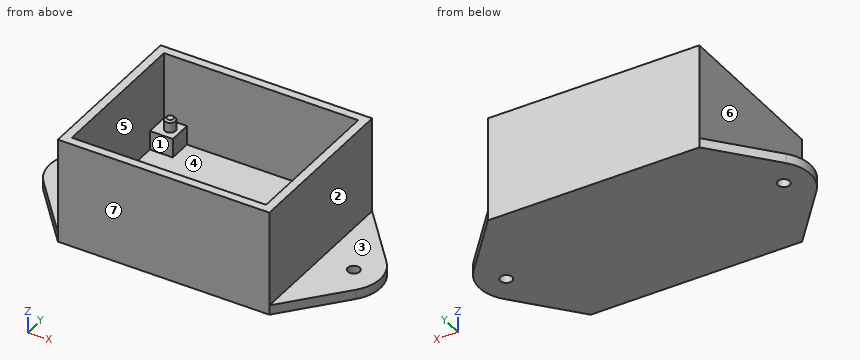
from build123d import *

# Parameters (mm, degrees)
F0_W      = 56.134
F0_H      = 44.45
F1_DEPTH  = 27.94
F2_W      = 51.562
F2_H      = 39.878
F3_DEPTH  = 22.86
F4_W      = 6.096
F4_H      = 6.096
F5_DEPTH  = 5.08
F6_R      = 1.397
F7_DEPTH  = 3.175
F8_SIZE   = 0.508
F10_DEPTH = 2.54
F11_R     = 1.5875
F12_DEPTH = 25.4


with BuildPart() as f1:
    # F0 (on Top) → F1 (new body)
    with BuildSketch(Plane.XY):
        Rectangle(F0_W, F0_H)
    extrude(amount=F1_DEPTH)

    # F2 (on face) → F3 (cut)
    with BuildSketch(Plane.XY.offset(27.94)):
        Rectangle(F2_W, F2_H)
    extrude(amount=-F3_DEPTH, mode=Mode.SUBTRACT)

    # F4 (on face) → F5 (join)
    with BuildSketch(Plane.XY.offset(5.08)):
        with Locations((-22.733, 16.891)):
            Rectangle(F4_W, F4_H)
        with Locations((22.733, 16.891)):
            Rectangle(F4_W, F4_H)
        with Locations((-22.733, -16.891)):
            Rectangle(F4_W, F4_H)
        with Locations((22.733, -16.891)):
            Rectangle(F4_W, F4_H)
    extrude(amount=F5_DEPTH)

    # F6 (on face) → F7 (join)
    with BuildSketch(Plane.XY.offset(10.16)):
        with Locations((-22.225, 16.85925)):
            Circle(F6_R)
        with Locations((22.225, 16.85925)):
            Circle(F6_R)
        with Locations((22.225, -16.85925)):
            Circle(F6_R)
        with Locations((-22.225, -16.85925)):
            Circle(F6_R)
    extrude(amount=F7_DEPTH)

    # F8
    f8_edges = [f1.edges().sort_by_distance(p)[0] for p in [
        (-23.622, 16.85925, 13.335),
        (20.828, 16.85925, 13.335),
        (-23.622, -16.85925, 13.335),
        (20.828, -16.85925, 13.335),
    ]]
    chamfer(f8_edges, length=F8_SIZE)

    # F9 (on face) → F10 (join)
    with BuildSketch(Plane(origin=(0, 0, 0), x_dir=(1, 0, 0), z_dir=(0, 0, -1))):
        with BuildLine():
            Line((41.449537, 6.61204), (28.067, 22.225))
            Line((28.067, 22.225), (28.067, -22.225))
            Line((28.067, -22.225), (41.449537, -6.61204))
            ThreePointArc((41.449537, -6.61204), (43.89549, 0), (41.449537, 6.61204))
        make_face()
        with BuildLine():
            Line((-28.067, -22.225), (-28.067, 22.225))
            Line((-28.067, 22.225), (-41.449537, 6.61204))
            ThreePointArc((-41.449537, 6.61204), (-43.89549, 0), (-41.449537, -6.61204))
            Line((-41.449537, -6.61204), (-28.067, -22.225))
        make_face()
    extrude(amount=-F10_DEPTH)

    # F11 (on face) → F12 (cut)
    with BuildSketch(Plane(origin=(0, 0, 0), x_dir=(1, 0, 0), z_dir=(0, 0, -1))):
        with Locations((-36.83, 0)):
            Circle(F11_R)
        with Locations((36.83, 0)):
            Circle(F11_R)
    extrude(amount=-F12_DEPTH, mode=Mode.SUBTRACT)


solid = f1.part
Input: part model. Units: mm. Frame: model coordinates. Face numbers are marked on the shaded views. A direction names the side the tool comes from. Coordinates: 2 decimals unless noted, no trailing zeros. Order: outer loops, then holes, each group sorted by start corner. A loop starts at its lowest first (then second) coordinate and runs counter-clockwise, first axis right, second up.
1. Access query for the marked faces 5, 6 and 7. Directions: +Z, -Z, +X, -X, +Y, -Y. A direction counts if a zero-diameter tool reaches every point of the face in a straight line with its end or side. Return the directions, or none.
Checked values:
face 5: +Z
face 6: +Z, -X, +Y, -Y
face 7: +Z, -Z, +X, -X, -Y
2. Draft query along X for the marked faces 1, 2, 3 and 4. Return one class per face: +X half, -X half, draft (parallel to the pull), parting line (faces both ways), or undercut.
Checked values:
face 1: undercut
face 2: +X half
face 3: draft
face 4: undercut
3. Cut plane C-C, the plane x = -5.5. Return loops of the section in (y, z) (3 decimals), plus the area to 3 significant figures.
Checked values:
outline: (-22.225, 0) - (22.225, 0) - (22.225, 27.94) - (19.939, 27.94) - (19.939, 5.08) - (-19.939, 5.08) - (-19.939, 27.94) - (-22.225, 27.94) - close
area: 330 mm2
4. Cut plane D-D, the plane x = 36.83. Return loops of the section in (y, z), plus the area to 3 significant figures.
Checked values:
outline: (-12, 0) - (-1.59, 0) - (-1.59, 2.54) - (-12, 2.54) - close; (1.59, 0) - (12, 0) - (12, 2.54) - (1.59, 2.54) - close
area: 52.9 mm2
5. Contact query for flat-ended pins moving along their axis: P1, Ø6, axis at y = -4.5, z = 23, coming from the -X side; P2, Ø5.5, axis at y = 18, z = 8, coming from the +X side; P3, Ø8, axis at x = 36.5, y = -2, coming from the +Z side. Output: stop coordinate, or through.
Checked values:
P1: stops at x = -28.07
P2: stops at x = 28.07
P3: stops at z = 2.54
6. Ray query, line 1 along X through (y, z) = (0, 0.9); line 2 along X through (y, z) = (-12, 25.5); line 3 along Y through (x, z) = (-19, 16.5) (3 decimals). Return the intervals inside material, ascending.
Checked values:
line 1: x = -43.9 to -38.42, -35.24 to 35.24, 38.42 to 43.9
line 2: x = -28.07 to -25.78, 25.78 to 28.07
line 3: y = -22.225 to -19.939, 19.939 to 22.225
7. Cut plane A-A, the plane z = 17.25. Return loops of the section in (x, y) (3 decimals), plus the area to 3 significant figures.
Checked values:
outline: (-28.067, -22.225) - (28.067, -22.225) - (28.067, 22.225) - (-28.067, 22.225) - close; hole (-25.781, -19.939) - (25.781, -19.939) - (25.781, 19.939) - (-25.781, 19.939) - close
area: 439 mm2
8. Cut plane B-B, the plane y = 0. Return loops of the section in (x, z), plus the area to 3 significant figures.
Checked values:
outline: (-43.9, 0) - (-38.42, 0) - (-38.42, 2.54) - (-43.9, 2.54) - close; (-35.24, 0) - (35.24, 0) - (35.24, 2.54) - (28.07, 2.54) - (28.07, 27.94) - (25.78, 27.94) - (25.78, 5.08) - (-25.78, 5.08) - (-25.78, 27.94) - (-28.07, 27.94) - (-28.07, 2.54) - (-35.24, 2.54) - close; (38.42, 0) - (43.9, 0) - (43.9, 2.54) - (38.42, 2.54) - close
area: 454 mm2
